Print and shaded views of the part. All mm, measured from the part's lowest x, y and z. Round coordinates to 2 decimals unless told otherwise and drop trailing zeros. Write each loop counter-clockwise with the first axis right and the second up, starting at its lowest first coordinate (ties: lowest second). Pieces come first, ordered by that corner, then holes.
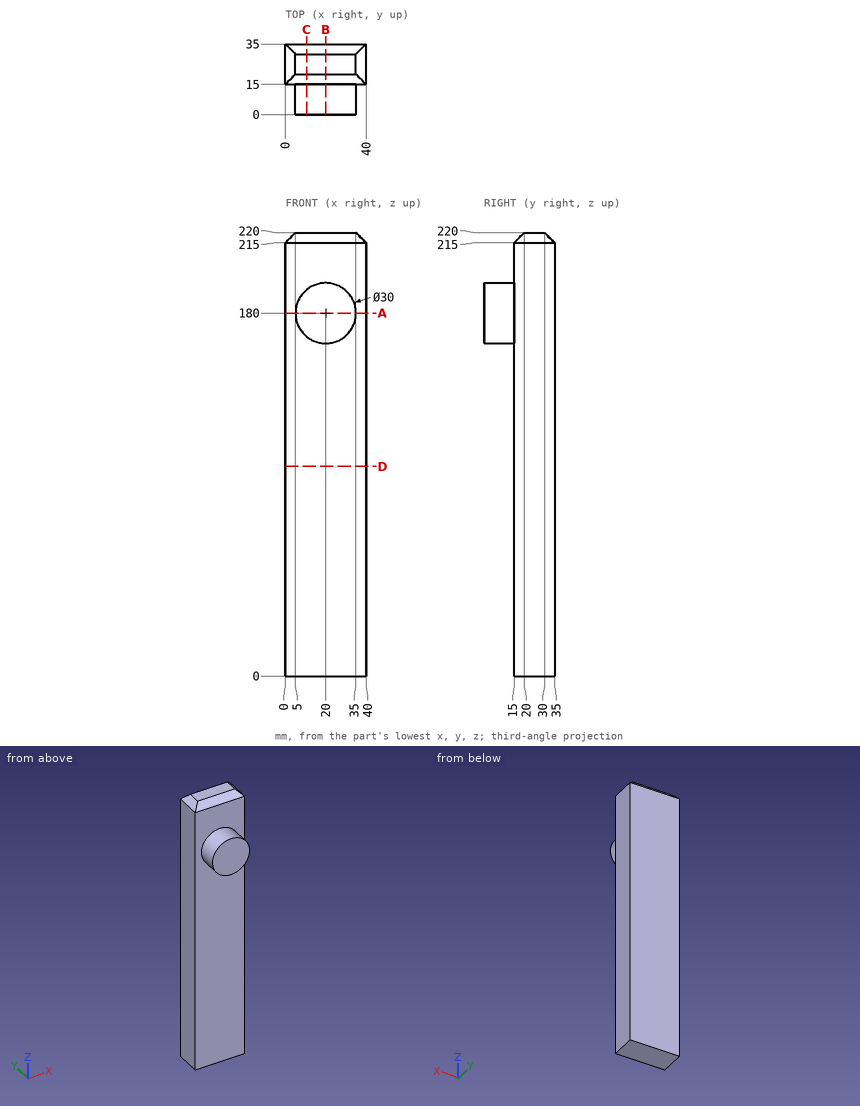
1) Slice it at A-A (z = 180). Write the cut outline in (x, y), plus the area to 3 significant figures.
Results:
outline: (0, 15) - (5, 15) - (5, 0) - (35, 0) - (35, 15) - (40, 15) - (40, 35) - (0, 35) - close
area: 1,250 mm2
2) Slice it at B-B (x = 20). Write the cut outline in (y, z), plus the area to 4 significant figures.
Results:
outline: (0, 165) - (15, 165) - (15, 0) - (35, 0) - (35, 215) - (30, 220) - (20, 220) - (15, 215) - (15, 195) - (0, 195) - close
area: 4,825 mm2
3) Slice it at C-C (x = 10.5). Write the cut outline in (y, z), plus the area to 3 significant figures.
Results:
outline: (0, 168.39) - (15, 168.39) - (15, 0) - (35, 0) - (35, 215) - (30, 220) - (20, 220) - (15, 215) - (15, 191.61) - (0, 191.61) - close
area: 4,720 mm2
4) Pin check, flat tips, straight feed: pin 1 Ø12 at (x, z) = (25.5, 58.5) entering from -Y; pin 2 Ø3 at (y, z) = (8, 166.5) entering from -X; pin 3 Ø1 at (x, y) = (32.5, 4.5) entering from +Z. Stop position of each tip, or through.
Results:
pin 1: stops at y = 15
pin 2: stops at x = 11
pin 3: stops at z = 189
5) Wall check: L1, parallel to Y at x = 5, z = 146; L2, parallel to Z at x = 2.5, y = 19; L3, parallel to Z at x = 32.5, y = 19. Give the ranges that are in metal, low to high.
Results:
L1: y = 15 to 35
L2: z = 0 to 217.5
L3: z = 0 to 219
6) Slice it at D-D (z = 104). Write the cut outline in (x, y).
Results:
outline: (0, 15) - (40, 15) - (40, 35) - (0, 35) - close
